Here's how the part is built. I have some questions about the finished solid (model axes, mm). A direction names the side the tool comes from. Coordinates: 2 decimals unless noted, no trailing zeros. Loops run counter-clockwise (first coordinate to the right, second up) from the corner with the lowest first, then second, coordinate; pieces in that order, holes last. Notation, with made-up numbers: (-26.5, 13.25) -> (27.5, 13.25) arc R16 cw to (27.5, 27.25) -> close; hole circle Ø8 at (-10.75, -26). An arc over 180 degrees is marked (long way). Answer as a JSON object with one key per item and string values. Group by question number.
1) I need wall thicknesses on probe 1 along Y at (x, z) = (-14, 2.35); probe 2 along Z at (x, y) = (-15, 12.5); probe 3 along Z at (x, y) = (-8.5, 11). Which ranges of each line are inside material? Lowest first, please. Write a range as [from, to].
2) I want a section at C-C (x = -20.5). Write out the boundary of the cut face in (y, z).
3) I want a section at B-B (y = 15). Write out the boundary of the cut face in (x, z).
4) I want a section at A-A (z = 1.25). Write out the boundary of the cut face in (x, y), then the cut area to 3 significant figures.
5) I'm going to push flat-ended pins straight in: pin 1 (0.6 mm diameter, centred on x = -13, z = 3, fed in from -Y); pin 2 (1 mm diameter, centred on y = 4, z = 2.5, fed in from +X); pin 3 (2 mm diameter, centred on x = -6, y = 10, fed in from +Z). Where does each tip first touch, or does it pass through?
6) Which directions (+Z, -Z, +X, -X, +Y, -Y) give clear straight access to the entire face, cutting with the end or side of a thin tool? Please do faces 1 (the flat face through (-13, 22.03, 3)), 2 (the flat face through (-11.632, 16.814, 2.614)), 3 (the flat face through (-8.882, 22.717, 2.614)), 4 (the flat face through (-18.434, 16, 3)).
7) If we mould it in two halves opening along Y, with no side actions, what happens to faces 5 (the flat face through (-9.84, 20.5, 2.6)), 6 (the flat face through (-19.373, 20.791, 2.614)), 7 (the flat face through (-6, 8, 2.6))? For each: +Y half, -Y half, draft (parallel to the pull), parting line (faces both ways), or undercut.
```python
from build123d import *

# Parameters (mm, degrees)
P_IDAT_VYSUNUT_M5_DEPTH = 1.6
P_IDAT_VYSUNUT_M6_DEPTH = 1
SKETCH1_W               = 14
SKETCH1_H               = 8.811343348
BOSS_EXTRUDE1_DEPTH     = 2
SKETCH2_W               = 14
SKETCH2_H               = 8.811343348
CUT_EXTRUDE1_DEPTH      = 2


with BuildPart() as part:
    # Skica1 → Přidat vysunutím5 (new body)
    with BuildSketch(Plane.XY):
        Polygon((0, 0), (0, 20), (-12.412784718, 31.615626352), (-23, 25), (-23, 0), align=None)
    extrude(amount=P_IDAT_VYSUNUT_M5_DEPTH)

    # Skica2 → Přidat vysunutím6 (add)
    with BuildSketch(Plane.XY.offset(1.6)):
        with BuildLine():
            Line((-3.705128205, 4.115384615), (-3.705128205, 2))
            Line((-3.705128205, 2), (-10.897435897, 2))
            add(Edge.make_bspline(
                [(-10.897435897, 2), (-10.87308441, 2.180790308), (-10.824395089, 2.542269551), (-10.673865117, 3.070299742), (-10.472959166, 3.585566992), (-10.254913916, 4.004869463), (-10.038043764, 4.342393523), (-9.841277463, 4.618963346), (-9.60654249, 4.913221767), (-9.337245105, 5.227544267), (-9.034873554, 5.562913411), (-8.697171951, 5.918082368), (-8.322529407, 6.291350846), (-8.058961705, 6.54481851), (-7.922676282, 6.67588141)],
                knots=[0, 0, 0, 0, 0.000546661, 0.001093015, 0.001642153, 0.002203944, 0.002507135, 0.00284526, 0.003221747, 0.003635945, 0.00408685, 0.004576261, 0.005106025, 0.00567326, 0.00567326, 0.00567326, 0.00567326], degree=3))
            add(Edge.make_bspline(
                [(-7.922676282, 6.67588141), (-7.813918956, 6.780862005), (-7.606877039, 6.980714138), (-7.312048947, 7.266894293), (-7.052864674, 7.529975199), (-6.823905036, 7.763139303), (-6.630459323, 7.972323552), (-6.469982936, 8.154242742), (-6.34044346, 8.309637702), (-6.270284768, 8.408220362), (-6.239182692, 8.451923077)],
                knots=[0, 0, 0, 0, 0.000453482, 0.000863296, 0.001232576, 0.001561374, 0.001843606, 0.002087173, 0.00228919, 0.002450062, 0.002450062, 0.002450062, 0.002450062], degree=3))
            add(Edge.make_bspline(
                [(-6.239182692, 8.451923077), (-6.175493233, 8.557718073), (-6.052643645, 8.761784362), (-5.91792888, 9.082682292), (-5.837068057, 9.403513936), (-5.825971765, 9.617891805), (-5.820512821, 9.723357372)],
                knots=[0, 0, 0, 0, 0.000370068, 0.000713818, 0.001040364, 0.001356575, 0.001356575, 0.001356575, 0.001356575], degree=3))
            add(Edge.make_bspline(
                [(-5.820512821, 9.723357372), (-5.824474653, 9.833108474), (-5.831970132, 10.040748999), (-5.894821019, 10.333768175), (-6.006276867, 10.585659667), (-6.15973106, 10.797196661), (-6.353774193, 10.962935085), (-6.580616259, 11.085399693), (-6.843577862, 11.153106661), (-7.028402789, 11.16201224), (-7.125, 11.166666667)],
                knots=[0, 0, 0, 0, 0.000329064, 0.000622563, 0.000892834, 0.001149779, 0.00139978, 0.001652148, 0.001916728, 0.002206405, 0.002206405, 0.002206405, 0.002206405], degree=3))
            add(Edge.make_bspline(
                [(-7.125, 11.166666667), (-7.220944609, 11.16231978), (-7.406288878, 11.153922533), (-7.669703299, 11.080565334), (-7.900142302, 10.953576306), (-8.06436539, 10.808860058), (-8.175305876, 10.668134018), (-8.250896853, 10.545500545), (-8.316050374, 10.406151312), (-8.37378183, 10.251655158), (-8.419383153, 10.080242168), (-8.456107626, 9.893217825), (-8.485702239, 9.689575671), (-8.495113848, 9.547907653), (-8.5, 9.474358974)],
                knots=[0, 0, 0, 0, 0.000287482, 0.000555353, 0.000811759, 0.001070877, 0.001205779, 0.00134826, 0.001502018, 0.001666561, 0.00184243, 0.002033439, 0.002238177, 0.002459233, 0.002459233, 0.002459233, 0.002459233], degree=3))
            Line((-8.5, 9.474358974), (-10.615384615, 9.681490385))
            add(Edge.make_bspline(
                [(-10.615384615, 9.681490385), (-10.598377251, 9.824305509), (-10.565402688, 10.101201217), (-10.483114114, 10.498918926), (-10.378898684, 10.865831465), (-10.247788098, 11.201257911), (-10.095201314, 11.507331251), (-9.913355139, 11.779458664), (-9.708603468, 12.020654551), (-9.480769352, 12.230790543), (-9.231301205, 12.410535137), (-8.969529148, 12.57098477), (-8.690337423, 12.702604473), (-8.396799939, 12.811078884), (-8.089049352, 12.897770766), (-7.765662274, 12.955090263), (-7.42863453, 12.995409017), (-7.198577984, 12.998446608), (-7.080929487, 13)],
                knots=[0, 0, 0, 0, 0.000431306, 0.000836233, 0.001217004, 0.001574233, 0.001915203, 0.002240945, 0.002553567, 0.002862328, 0.003168197, 0.003474678, 0.003782194, 0.004092453, 0.004412693, 0.004739863, 0.005076887, 0.005429623, 0.005429623, 0.005429623, 0.005429623], degree=3))
            add(Edge.make_bspline(
                [(-7.080929487, 13), (-6.953030371, 12.997541845), (-6.703930784, 12.992754281), (-6.34028961, 12.953218534), (-5.998674853, 12.884282231), (-5.676099879, 12.79296634), (-5.375877361, 12.67105295), (-5.095505554, 12.52366473), (-4.83939702, 12.345207999), (-4.603734114, 12.145414763), (-4.393070332, 11.925706984), (-4.20854792, 11.691351493), (-4.053955652, 11.442511564), (-3.924228998, 11.182220281), (-3.827907833, 10.90628918), (-3.757724044, 10.618533633), (-3.711189366, 10.317611197), (-3.707170936, 10.112088), (-3.705128205, 10.007612179)],
                knots=[0, 0, 0, 0, 0.000383641, 0.00074719, 0.0010955, 0.001428145, 0.001751403, 0.002065859, 0.002376361, 0.002685876, 0.002991333, 0.003287991, 0.003579024, 0.003868752, 0.004158681, 0.00445369, 0.004756592, 0.005069772, 0.005069772, 0.005069772, 0.005069772], degree=3))
            add(Edge.make_bspline(
                [(-3.705128205, 10.007612179), (-3.707819477, 9.887707131), (-3.713158546, 9.649833916), (-3.764276175, 9.298186238), (-3.84237396, 8.954647512), (-3.957796338, 8.618378159), (-4.104103161, 8.28131186), (-4.292696164, 7.942692037), (-4.511666905, 7.592306518), (-4.683112364, 7.36576699), (-4.771634615, 7.248798077)],
                knots=[0, 0, 0, 0, 0.000359506, 0.000713204, 0.001063842, 0.00141504, 0.001778167, 0.002164709, 0.002576738, 0.003016589, 0.003016589, 0.003016589, 0.003016589], degree=3))
            add(Edge.make_bspline(
                [(-4.771634615, 7.248798077), (-4.80509214, 7.206658226), (-4.876750403, 7.116404431), (-4.998659939, 6.978014195), (-5.139942605, 6.826848432), (-5.298602846, 6.660077667), (-5.479881522, 6.483607708), (-5.677256214, 6.290058721), (-5.899411985, 6.089331377), (-6.12951153, 5.876418507), (-6.360611244, 5.669193404), (-6.5730252, 5.472375498), (-6.765967752, 5.298233923), (-6.930453202, 5.137155265), (-7.076156545, 5.000133027), (-7.197826149, 4.880140867), (-7.29773874, 4.780083699), (-7.43541186, 4.624119958), (-7.610585282, 4.413178934), (-7.733826947, 4.21161882), (-7.792668269, 4.115384615)],
                knots=[0, 0, 0, 0, 0.0001614, 0.000345681, 0.000553058, 0.000782151, 0.00103613, 0.001311959, 0.001611379, 0.001934216, 0.002252456, 0.002542536, 0.002802971, 0.003032064, 0.003233117, 0.00340296, 0.003544758, 0.003657116, 0.004027059, 0.004365069, 0.004365069, 0.004365069, 0.004365069], degree=3))
            Line((-7.792668269, 4.115384615), (-3.705128205, 4.115384615))
        make_face()
    extrude(amount=P_IDAT_VYSUNUT_M6_DEPTH)

    # Sketch1 → Boss-Extrude1 (add)
    with BuildSketch(Plane.XY.offset(1.6)):
        with Locations((-14, 19.405671674)):
            Rectangle(SKETCH1_W, SKETCH1_H)
    extrude(amount=BOSS_EXTRUDE1_DEPTH)

    # Sketch2 → Cut-Extrude1 (cut)
    with BuildSketch(Plane.XY.offset(3.6)):
        with Locations((-14, 19.405671674)):
            Rectangle(SKETCH2_W, SKETCH2_H)
        Polygon((-19.444720722, 20.35888782), (-19.444720722, 19.986569127), (-19.131189191, 19.418293227), (-19.131189191, 18.066188499), (-19.131189191, 17.772252689), (-18.858242416, 17.277536659), (-18.858242416, 15.342383323), (-18.288573201, 15.518744809), (-18.433763737, 15.781902655), (-18.433763737, 16.890445258), (-17.976410423, 17.14277812), (-17.446333305, 15.430564066), (-16.936468473, 15.430564066), (-17.049096134, 15.794365214), (-17.191400889, 17.277536659), (-17.191400889, 17.524894674), (-16.936468473, 17.665547041), (-16.936468473, 17.919220594), (-16.426979735, 17.792383818), (-15.689001428, 17.608664763), (-13.526813072, 17.608664763), (-13.06092643, 17.14277812), (-13.293869751, 15.430564066), (-12.547027038, 15.430564066), (-12.747744912, 15.794365214), (-12.747744912, 16.286671093), (-12.547027038, 17.14277812), (-12.253091227, 17.14277812), (-12.253091227, 15.430564066), (-11.430070958, 15.430564066), (-11.697847079, 16.040518153), (-11.563959019, 17.608664763), (-10.856559128, 17.919220594), (-10.430689203, 18.458102913), (-10.293165377, 19.044673063), (-10.019179068, 19.614250434), (-9.840080969, 19.986569127), (-9.840080969, 20.574440748), (-9.840080969, 21.044738045), (-9.705647537, 21.221099531), (-9.431307447, 21.221099531), (-9.254945961, 21.221099531), (-9.023579601, 21.044738045), (-8.627882899, 21.044738045), (-8.427020311, 21.132918788), (-8.275159926, 21.221099531), (-8.09879844, 21.221099531), (-7.981224116, 21.397461017), (-7.981224116, 21.652205386), (-8.348696256, 22.285047188), (-9.431307447, 23.161851588), (-9.705647537, 23.344744981), (-10.64624213, 23.344744981), (-11.128859966, 23.064503366), (-11.697847079, 22.457055221), (-12.098019445, 22.02983296), (-12.547027038, 22.02983296), (-14.03630181, 22.02983296), (-17.661510139, 22.24344409), (-18.61604593, 21.824393055), (-19.008263773, 21.652205386), (-19.30233871, 21.21109298), align=None, mode=Mode.SUBTRACT)
    extrude(amount=-CUT_EXTRUDE1_DEPTH, mode=Mode.SUBTRACT)


solid = part.part
```
Determined:
{
 "1": {"probe 1": "[17.61, 22.03]", "probe 2": "[0, 1.6]", "probe 3": "[0, 2.6]"},
 "2": {"outline": "(0, 0) -> (26.56, 0) -> (26.56, 1.6) -> (0, 1.6) -> close"},
 "3": {"outline": "(-23, 0) -> (0, 0) -> (0, 1.6) -> (-23, 1.6) -> close"},
 "4": {"outline": "(-23, 0) -> (0, 0) -> (0, 20) -> (-12.41, 31.62) -> (-23, 25) -> close", "area": "620 mm^2"},
 "5": {"pin 1": "y = 15.43", "pin 2": "x = -3.71", "pin 3": "z = 2.6"},
 "6": {"face 1": "+Z, +Y", "face 2": "+Z, +X", "face 3": "+Z, +X, +Y", "face 4": "+Z"},
 "7": {"face 5": "undercut", "face 6": "+Y half", "face 7": "draft"}
}
